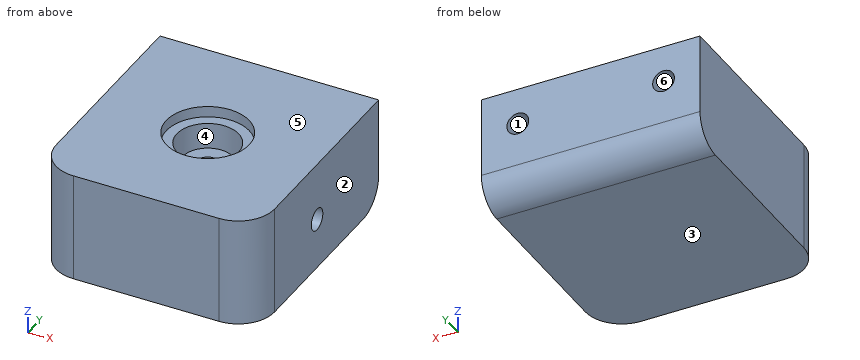
from build123d import *

# Parameters (mm, degrees)
F0_W      = 38.1
F0_H      = 40.64
F1_DEPTH  = 19.05
F4_R      = 7.239
F5_DEPTH  = 1.905
F6_R      = 6.35
F8_R      = 1.89865
F10_R     = 1.89865
F11_DEPTH = 12.7
F12_R     = 5.08


with BuildPart() as f1:
    # F0 (on Top) → F1 (new body)
    with BuildSketch(Plane.XY):
        Rectangle(F0_W, F0_H)
    extrude(amount=-F1_DEPTH)

    # F2 (on Front) → F3 (revolve, cut)
    with BuildSketch(Plane.XZ):
        Polygon((5.3975, 0), (0, 0), (0, -5.7912), (4.3815, -5.7912), (4.3815, -7.0612), (5.3975, -7.0612), align=None)
    revolve(axis=Axis((0, 0, -9.525), (0, 0, -1)), mode=Mode.SUBTRACT)

    # F4 (on face) → F5 (cut)
    with BuildSketch(Plane.XY):
        Circle(F4_R)
    extrude(amount=-F5_DEPTH, mode=Mode.SUBTRACT)

    # F6
    f6_edges = [f1.edges().sort_by_distance(p)[0] for p in [
        (-19.05, -20.32, -9.525),
        (19.05, -20.32, -9.525),
    ]]
    fillet(f6_edges, radius=F6_R)

    # F9: sweep along a path in F7
    with BuildLine(Plane.XZ) as f9_path:
        Line((0, -5.7912), (0, -7.62))
        ThreePointArc((0, -7.62), (0.7439487758, -9.4160512242), (2.54, -10.16))
        Line((2.54, -10.16), (19.05, -10.16))
    # F8 (on face) → F9 (sweep, cut)
    with BuildSketch(Plane.XY.offset(-5.7912)):
        Circle(F8_R)
    sweep(path=f9_path.line, mode=Mode.SUBTRACT)

    # F10 (on face) → F11 (cut)
    with BuildSketch(Plane(origin=(0, 20.32, 0), x_dir=(-1, 0, 0), z_dir=(0, 1, 0))):
        with Locations((-12.7, -6.35)):
            Circle(F10_R)
        with Locations((12.7, -6.35)):
            Circle(F10_R)
    extrude(amount=-F11_DEPTH, mode=Mode.SUBTRACT)

    # F12
    f12_edges = [f1.edges().sort_by_distance(p)[0] for p in [
        (0, 20.32, -19.05),
    ]]
    fillet(f12_edges, radius=F12_R)


solid = f1.part
Verification items for the finished model (mm, model axes). Face numbers are marked on the shaded views. A direction names the side the tool comes from. Coordinates: 2 decimals unless noted, no trailing zeros. Order: outer loops, then holes, each group sorted by start corner. A loop starts at its lowest first (then second) coordinate and runs counter-clockwise, first axis right, second up. Notation, with made-up numbers: M 4,-3.75 L 21,-3.75 A24 ccw 21,9.25 Z; hole C 86,51 d4. An arc over 180 degrees is marked long. Write each question's results on one line, items separated by ' | '.
1) Access from +Z, -Z, +X, -X, +Y, -Y to the whole of each face (thin tool, end or side, straight path). Record for the marked faces 4, 5 and 6.
Solved:
face 4: +Z | face 5: +Z, +X, -X, +Y, -Y | face 6: +Y
2) Section check C-C on z = -15.5. Record the cut outline in (x, y).
Solved:
outline: M -19.05,-13.97 A6.35 ccw -12.7,-20.32 L 12.7,-20.32 A6.35 ccw 19.05,-13.97 L 19.05,20.08 L -19.05,20.08 Z
3) Section check D-D on x = -6.5. Record the cut outline in (y, z) (3 decimals).
Solved:
outline: M -20.32,-19.05 L 15.24,-19.05 A5.08 ccw 20.32,-13.97 L 20.32,0 L 3.186,0 L 3.186,-1.905 L -3.186,-1.905 L -3.186,0 L -20.32,0 Z
4) Release check for a two-part mould opening along Z. For the marked faces 1, 2 and 3 record: pulls with the +Z half, pulls with the -Z half, needs draft (parallel to the pull), parting line crosses it, or undercut.
Solved:
face 1: undercut | face 2: needs draft | face 3: pulls with the -Z half
5) Section check B-B on x = -11.5. Record the cut outline in (y, z).
Solved:
outline: M -20.32,-19.05 L 15.24,-19.05 A5.08 ccw 20.32,-13.97 L 20.32,-7.82 L 7.62,-7.82 L 7.62,-4.88 L 20.32,-4.88 L 20.32,0 L -20.32,0 Z
6) Scan lines: line 1 along Y through (x, z) = (0, -7); line 2 along X through (y, z) = (0, -6.5); line 3 along X through (y, z) = (0, -3.85). Record each from-to range of solid material in increasing order. Write a range as [from, to].
Solved:
line 1: y = [-20.32, -5.4], [-4.38, -1.9], [1.9, 4.38], [5.4, 20.32] | line 2: x = [-19.05, -5.4], [-4.38, -1.9], [1.9, 4.38], [5.4, 19.05] | line 3: x = [-19.05, -5.4], [5.4, 19.05]
7) Gauge pin test, flat ends, axial feed: pin 1 Ø10 at (x, z) = (-13.5, -8) entering from -Y; pin 2 Ø13 at (x, y) = (0, 0) entering from +Z (3 decimals); pin 3 Ø5.5 at (x, y) = (-1.5, -2) entering from +Z; pin 4 Ø3 at (x, z) = (-12.5, -6.5) entering from +Y. Record the tip position at first contact, or that the pin passes through.
Solved:
pin 1: stops at y = -20.32 | pin 2: stops at z = -1.905 | pin 3: stops at z = -5.79 | pin 4: stops at y = 7.62
